Build history of the part. All positions in model axes, mm. Face numbers are marked on the shaded views. A direction names the side the tool comes from. Round coordinates to 2 decimals unless told otherwise and drop trailing zeros. Order: outer loops, then holes, each group sorted by start corner. A loop starts at its lowest first (then second) coordinate and runs counter-clockwise, first axis right, second up. Notation, with made-up numbers: (33.25, -26.75) -> (76.25, -26.75) arc R18 cw to (76.25, -3.75) -> close; hole circle Ø2 at (-1.75, -33.5). An arc over 180 degrees is marked (long way). Answer as a JSON object with one key per item and string values.
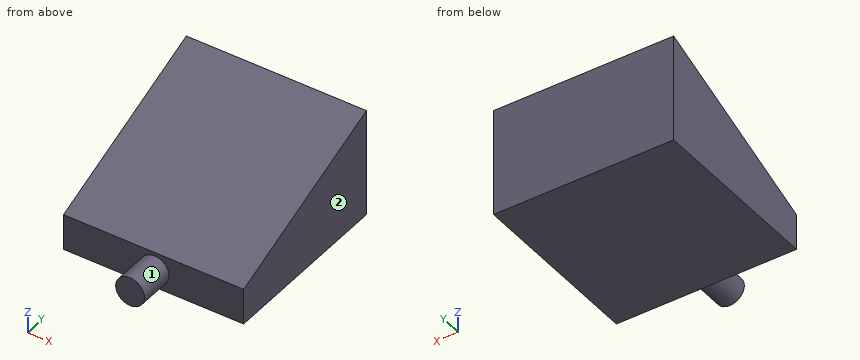
from build123d import *

# Parameters (mm, degrees)
F0_W     = 114.1541988105
F0_H     = 25.4
F1_DEPTH = 127
F2_R     = 10.16
F3_DEPTH = 25.4


# Not quite as in the source:
# - a feature names something its author has since deleted; it is built from what else it names


with BuildPart() as f1:
    # F0 (on Right) → F1 (new body)
    with BuildSketch(Plane.YZ):
        Polygon((127, 63.5), (0, 12.7), (12.8458011895, 12.7), (127, 12.7), align=None)
        with Locations((69.9229005948, 0)):
            Rectangle(F0_W, F0_H)
        Polygon((12.8458011895, 12.7), (0, 12.7), (0, 0), (0, -12.7), (12.8458011895, -12.7), align=None)
    extrude(amount=F1_DEPTH)

    # F2 (on face) → F3 (join)
    with BuildSketch(Plane.XZ):
        with Locations((64.2495304346, 0)):
            Circle(F2_R)
    extrude(amount=F3_DEPTH)


solid = f1.part
1) Probe L1, parallel to Y at x = 33, z = 2; L2, parallel to Z at x = 38, y = 63.5; L3, parallel to Z at x = 9, y = 61. List the from-to ranges inside material, lowest first. Write a range as from..to.
Checked values:
{"L1": "y = 0..127", "L2": "z = -12.7..38.1", "L3": "z = -12.7..37.1"}
2) Flat gauge pins, fed straight in: pin 1 Ø1 at (x, z) = (24.5, 3) entering from -Y; pin 2 Ø10 at (x, y) = (84.5, 37) entering from +Z; pin 3 Ø8 at (x, z) = (14.5, 41.5) entering from -Y. Where does each tip first touch, or does it go through?
Checked values:
{"pin 1": "stops at y = 0", "pin 2": "stops at z = 29.5", "pin 3": "stops at y = 62"}
3) Cut at A-A, the plane z = 0. Give the cut face in (x, y).
Checked values:
{"outline": "(0, 0) -> (54.09, 0) -> (54.09, -25.4) -> (74.41, -25.4) -> (74.41, 0) -> (127, 0) -> (127, 127) -> (0, 127) -> close"}
4) Which spindle directions (+Z, -Z, +X, -X, +Y, -Y) get a long thin tool onto all of the face, cutting with end or side? Do the marked faces 1 and 2. Say none if no direction does.
Checked values:
{"face 1": "-Y", "face 2": "+Z, -Z, +X, +Y, -Y"}
5) Cut at C-C, the plane y = 72. Give the cut face in (x, z).
Checked values:
{"outline": "(0, -12.7) -> (127, -12.7) -> (127, 41.5) -> (0, 41.5) -> close"}
6) Cut at B-B, the plane x = 46. Give the cut face in (y, z), plus the area to 3 significant figures.
Checked values:
{"outline": "(0, -12.7) -> (127, -12.7) -> (127, 63.5) -> (0, 12.7) -> close", "area": "6,450 mm²"}
